Autodesk Inventor part; units mm, degrees
ref_plane "YZ Plane" through (0, 0, 0) normal (1, 0, 0) x (0, 1, 0)
ref_plane "XZ Plane" through (0, 0, 0) normal (0, 1, 0) x (-1, 0, 0)
ref_plane "XY Plane" through (0, 0, 0) normal (0, 0, 1) x (1, 0, 0)
sketch "Sketch1" plane through (0, 0, 0) normal (0, 0, 1) x (1, 0, 0)
  line L0 (0, 33.8) -> (12.5, 33.8)
  line L1 (12.5, 33.8) -> (12.5, 47.9)
  line L2 (12.5, 47.9) -> (91.4, 47.9)
  line L3 (91.4, 47.9) -> (91.4, -47.9)
  line L4 (91.4, -47.9) -> (12.5, -47.9)
  line L5 (12.5, -47.9) -> (12.5, -33.8)
  line L6 (12.5, -33.8) -> (0, -33.8)
  line L7 (0, -33.8) -> (0, 33.8)
  line L8 (-4.5, 48) -> (91.5, 48) construction
  line L9 (91.5, 48) -> (91.5, -48) construction
  line L10 (91.5, -48) -> (-4.5, -48) construction
  line L11 (-4.5, -48) -> (-4.5, 48) construction
  line L12 (-4.4, 47.9) -> (-3.4, 47.9) construction
  line L13 (-3.4, 47.9) -> (-3.4, -47.9) construction
  line L14 (-3.4, -47.9) -> (-4.4, -47.9) construction
  line L15 (-4.4, -47.9) -> (-4.4, 47.9) construction
  point P0 (0, 0)
  point P1 (0, 0)
  point P2 (-4.5, 0)
  dimension "d0" = 67.6
  dimension "d1" = 95.8
  dimension "d2" = 91.4
  dimension "d3" = 12.5
  dimension "d20" = 96
  dimension "d21" = 96
  dimension "d22" = 0.1
  dimension "d23" = 0.1
  dimension "d24" = 1
  dimension "d25" = 0.1
  dimension "d26" = 3.4
extrude "Extrusion1" add sketch "Sketch1" along normal mid plane 1
sketch "Sketch2" plane through (0, 0, 0.5) normal (0, 0, 1) x (1, 0, 0)
  line L0 (12.5, 33.8) -> (0, 33.8)
  line L1 (0, 33.8) -> (0, -33.8)
  line L2 (0, -33.8) -> (12.5, -33.8)
  line L3 (12.5, -33.8) -> (12.5, -47.9)
  line L4 (12.5, -47.9) -> (91.4, -47.9)
  line L5 (91.4, -47.9) -> (91.4, 47.9)
  line L6 (91.4, 47.9) -> (12.5, 47.9)
  line L7 (12.5, 47.9) -> (12.5, 33.8)
  line L8 (91.4, -47.9) -> (91.4, 47.9)
  line L9 (12.5, 47.9) -> (91.4, 47.9)
  line L10 (91.4, 47.9) -> (91.4, 45.4)
  line L11 (91.4, 45.4) -> (12.5, 45.4)
  line L12 (12.5, 45.4) -> (12.5, 47.9)
  line L13 (91.4, -47.9) -> (12.5, -47.9)
  line L14 (12.5, -47.9) -> (12.5, -45.4)
  line L15 (12.5, -45.4) -> (91.4, -45.4)
  line L16 (91.4, -45.4) -> (91.4, -47.9)
  point P0 (0, 0)
  dimension "d6" = 2.5
  dimension "d27" = 90.8
extrude "Extrusion2" add sketch "Sketch2" along normal blind 0.01 contours L7 L6 L5 L11 | L5 L4 L3 L15
mirror "Mirror1" about plane through (0, 0, 0) normal (0, 0, 1) of "Extrusion2"
sketch "Sketch3" plane through (0, 0, 0.5) normal (0, 0, 1) x (1, 0, 0)
  circle A0 centre (6, 31.8) radius 0.9
  circle A1 centre (6, -31.8) radius 0.9
  point P0 (0, 0)
  dimension "d9" = 1.8
  dimension "d10" = 6
  dimension "d11" = 31.8
  dimension "d12" = 31.8
extrude "Extrusion3" cut sketch "Sketch3" against normal through all
sketch "Sketch4" plane through (0, 0, 0.5) normal (0, 0, 1) x (1, 0, 0)
  circle A0 centre (6, 31.8) radius 0.9
  circle A1 centre (6, -31.8) radius 0.9
  line L0 (12.5, -45.4) -> (91.4, -45.4)
  line L1 (91.4, -45.4) -> (91.4, 45.4)
  line L2 (91.4, 45.4) -> (12.5, 45.4)
  line L3 (12.5, 45.4) -> (12.5, 33.8)
  line L4 (12.5, 33.8) -> (0, 33.8)
  line L5 (0, 33.8) -> (0, -33.8)
  line L6 (0, -33.8) -> (12.5, -33.8)
  line L7 (12.5, -33.8) -> (12.5, -45.4)
  line L8 (0, 18.95) -> (3.5, 18.95)
  arc A2 (3.5, 17.95) -> (3.5, 18.95) centre (3.5, 18.45) ccw
  line L9 (3.5, 17.95) -> (0, 17.95)
  point P0 (0, 0)
  dimension "d15" = 17.95
  dimension "d16" = 3.5
  dimension "d17" = 1
extrude "Extrusion4" cut sketch "Sketch4" against normal through all contours L5 L8 A2 L9
sketch "Sketch5" plane through (0, 0, 0.5) normal (0, 0, 1) x (1, 0, 0)
  line L0 (0, 18.95) -> (3.5, 18.95)
  arc A0 (3.5, 17.95) -> (3.5, 18.95) centre (3.5, 18.45) ccw
  line L1 (3.5, 17.95) -> (0, 17.95)
  line L2 (0, 17.95) -> (0, -33.8)
  line L3 (0, -33.8) -> (12.5, -33.8)
  line L4 (12.5, -33.8) -> (12.5, -45.4)
  line L5 (12.5, -45.4) -> (91.4, -45.4)
  line L6 (91.4, -45.4) -> (91.4, 45.4)
  line L7 (91.4, 45.4) -> (12.5, 45.4)
  line L8 (12.5, 45.4) -> (12.5, 33.8)
  line L9 (12.5, 33.8) -> (0, 33.8)
  line L10 (0, 33.8) -> (0, 18.95)
  circle A1 centre (6, -31.8) radius 0.9
  circle A2 centre (6, 31.8) radius 0.9
  circle A3 centre (43.4, 0) radius 6 construction
  line L11 (36.9, 12.5) -> (49.9, 12.5)
  line L12 (51.9, 10.5) -> (51.9, -10.5)
  line L13 (49.9, -12.5) -> (36.9, -12.5)
  line L14 (34.9, -10.5) -> (34.9, 10.5)
  arc A4 (36.9, 12.5) -> (34.9, 10.5) centre (36.9, 10.5) ccw
  arc A5 (51.9, 10.5) -> (49.9, 12.5) centre (49.9, 10.5) ccw
  arc A6 (49.9, -12.5) -> (51.9, -10.5) centre (49.9, -10.5) ccw
  arc A7 (34.9, -10.5) -> (36.9, -12.5) centre (36.9, -10.5) ccw
  point P0 (0, 0)
  point P1 (51.9, -12.5)
  point P2 (51.9, 12.5)
  point P3 (34.9, -12.5)
  point P4 (43.4, 12.5)
  point P5 (34.9, 0)
  dimension "d28" = 43.4
  dimension "d29" = 12
  dimension "d41" = 17
  dimension "d42" = 25
  dimension "d43" = 2
extrude "Extrusion5" cut sketch "Sketch5" against normal through all contours L11 A5 L12 A6 L13 A7 L14 A4
sketch "Sketch6" plane through (0, 0, 0.5) normal (0, 0, 1) x (1, 0, 0)
  line L0 (32.4, 10) -> (32.4, -10) construction
  circle A0 centre (43.4, 0) radius 6 construction
  point P0 (0, 0)
  point P1 (32.4, 0)
  dimension "d32" = 20
  dimension "d44" = 11
hole "Hole1" at (32.4, 10, 0.5) at (32.4, -10, 0.5) direction (0, 0, -1) diameter 2.2 end through all
equation "\"d23\" = d22"
equation "\"d25\" = d22"
properties part number "Payload_PCB" material "Epoxy Resin"
Source: CAD feature listing. Evaluate the final solid. Frame: model axes, mm. A direction names the side the tool comes from. Round coordinates to 2 decimals unless told otherwise and drop trailing zeros. Loops run counter-clockwise (first coordinate to the right, second up) from the corner with the lowest first, then second, coordinate; pieces in that order, holes last. Notation, with made-up numbers: (-33.75, -20) - (19.25, -20) arc R31 ccw to (19.25, 11) - close; hole circle Ø11 at (-30.75, -19). An arc over 180 degrees is marked (long way). Write item = value, one per line. Start each with the question number.
(1) Pull-direction query (Y, two-part tool) for faces 3 (the face through (51, -47, 0.51)), 4 (the face through (51.3, -11.93, 0.01)); classes: +Y half, -Y half, draft (parallel to the pull), parting line (faces both ways), or undercut.
(2) Set-up query: faces 1 (the face through (35.5, 11.93, 0.01)), 2 (the face through (55, 1, -0.5)). Return all of +Z, -Z, +X, -X, +Y, -Y with unobstructed straight access to the full face (end or side cutting, diameter ignored); none if empty.
(3) Section query B-B, the plane y = 1.5. Output: boundary loops of the cut face in (x, z), plus the area to 3 significant figures.
(4) Pin query (flat end, axial travel): pin 1 (5 mm diameter, centred on x = 33, y = -2, fed in from -Z); pin 2 (6 mm diameter, centred on x = 12, y = 4.5, fed in from +Z). Return the tip coordinate at first contact, or that it passes through.
(5) Section query C-C, the plane z = -0.1. Output: boundary loops of the cut face in (x, y).
(6) Ray query, line 1 along X through (y, z) = (-10, 0.3); line 2 along Y through (x, z) = (32.4, 0.3); line 3 along Y through (x, z) = (6, -0.2). Return the intervals inside material, ascending. Write a range as from..to.
Conclusion:
q1.face_3 = draft
q1.face_4 = undercut
q2.face_1 = +Z, -Z
q2.face_2 = -Z, +X, -X, +Y, -Y
q3.outline = (0, -0.5) - (34.9, -0.5) - (34.9, 0.5) - (0, 0.5) - close; (51.9, -0.5) - (91.4, -0.5) - (91.4, 0.5) - (51.9, 0.5) - close
q3.area = 74.4 mm2
q4.pin_1 = -0.5
q4.pin_2 = 0.5
q5.outline = (0, -33.8) - (12.5, -33.8) - (12.5, -47.9) - (91.4, -47.9) - (91.4, 47.9) - (12.5, 47.9) - (12.5, 33.8) - (0, 33.8) - (0, 18.95) - (3.5, 18.95) arc R0.5 cw to (3.5, 17.95) - (0, 17.95) - close; hole circle Ø1.8 at (6, -31.8); hole circle Ø1.8 at (6, 31.8); hole circle Ø2.2 at (32.4, -10); hole circle Ø2.2 at (32.4, 10); hole (34.9, -10.5) arc R2 ccw to (36.9, -12.5) - (49.9, -12.5) arc R2 ccw to (51.9, -10.5) - (51.9, 10.5) arc R2 ccw to (49.9, 12.5) - (36.9, 12.5) arc R2 ccw to (34.9, 10.5) - close
q6.line_1 = 0..31.3, 33.5..34.9, 51.9..91.4
q6.line_2 = -47.9..-11.1, -8.9..8.9, 11.1..47.9
q6.line_3 = -33.8..-32.7, -30.9..30.9, 32.7..33.8
